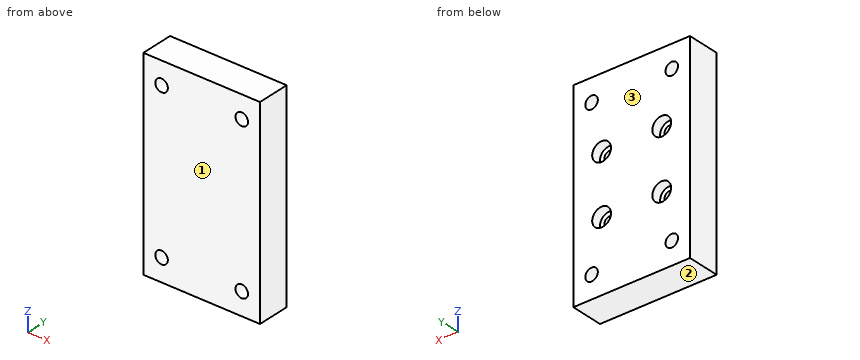
from build123d import *

# Parameters (mm, degrees)
SKETCH1_W                                       = 59.1185
SKETCH1_H                                       = 101.6
BOSS_EXTRUDE1_DEPTH                             = 16.51
CBORE_FOR_10_SOCKET_HEAD_CAP_SCREW1_D           = 5.1054
CBORE_FOR_10_SOCKET_HEAD_CAP_SCREW1_DEPTH       = 15.24
CBORE_FOR_10_SOCKET_HEAD_CAP_SCREW1_CBORE_D     = 9.525
CBORE_FOR_10_SOCKET_HEAD_CAP_SCREW1_CBORE_DEPTH = 4.826
F_1_4_0_25_DIAMETER_HOLE1_D                     = 6.35


with BuildPart() as part:
    # Sketch1 → Boss-Extrude1 (new body)
    with BuildSketch(Plane(origin=(0, 0, 0), x_dir=(1, 0, 0), z_dir=(0, 1, 0))):
        Rectangle(SKETCH1_W, SKETCH1_H)
    extrude(amount=BOSS_EXTRUDE1_DEPTH)

    # CBORE for #10 Socket Head Cap Screw1
    with Locations(Plane(origin=(-223.3968133, 16.51, 0), x_dir=(0, 0, 1), z_dir=(0, 1, 0))):
        with Locations((-14.986, 208.1568133), (14.986, 208.1568133), (14.986, 238.6368133), (-14.986, 238.6368133)):
            CounterBoreHole(CBORE_FOR_10_SOCKET_HEAD_CAP_SCREW1_D / 2, CBORE_FOR_10_SOCKET_HEAD_CAP_SCREW1_CBORE_D / 2, CBORE_FOR_10_SOCKET_HEAD_CAP_SCREW1_CBORE_DEPTH, depth=CBORE_FOR_10_SOCKET_HEAD_CAP_SCREW1_DEPTH)

    # 1/4 (0.25) Diameter Hole1 (through all)
    with Locations(Plane(origin=(0, 16.51, 0), x_dir=(1, 0, 0), z_dir=(0, 1, 0))):
        with Locations((20.32, -39.37), (-20.32, -39.37), (-20.32, 39.37), (20.32, 39.37)):
            Hole(F_1_4_0_25_DIAMETER_HOLE1_D / 2)


solid = part.part
Source: CAD feature listing. Evaluate the final solid. Frame: model axes, mm. Face numbers are marked on the shaded views. Give positions to 0.01 mm unless a question says otherwise; leave off trailing zeros. Order: outer loops, then holes, each group sorted by start corner. A loop starts at its lowest first (then second) coordinate and runs counter-clockwise, first axis right, second up. Notation, with made-up numbers: (46.25, 68.25) -> (100.25, 68.25) arc R27 cw to (100.25, 95.25) -> close; hole circle Ø4 at (36, 87.5). An arc over 180 degrees is marked (long way). Write item = value, one per line.
Item 1: Mould query, pull axis Y, two halves, no side actions, for the marked faces 1, 2 and 3. Classes: +Y half, -Y half, draft (parallel to the pull), parting line (faces both ways), or undercut.
Check result:
face_1 = -Y half
face_2 = draft
face_3 = +Y half
Item 2: Section query C-C (x = -21). Output: boundary loops of the cut face in (y, z), then the cut area to 3 significant figures.
Check result:
outline = (0, -50.8) -> (16.51, -50.8) -> (16.51, -42.47) -> (0, -42.47) -> close; (0, -36.27) -> (16.51, -36.27) -> (16.51, 36.27) -> (0, 36.27) -> close; (0, 42.47) -> (16.51, 42.47) -> (16.51, 50.8) -> (0, 50.8) -> close
area = 1,470 mm²
Item 3: Ray query, probe 1 along Z at (x, y) = (15, 8.5); probe 2 along X at (y, z) = (7, -39.37) (3 decimals); probe 3 along X at (y, z) = (14.25, -38.5). Return the intervals inside material, ascending.
Check result:
probe_1 = -50.8 to -17.53, -12.44 to 12.44, 17.53 to 50.8
probe_2 = -29.559 to -23.495, -17.145 to 17.145, 23.495 to 29.559
probe_3 = -29.56 to -23.37, -17.27 to 17.27, 23.37 to 29.56
Item 4: Section query A-A (y = 8.25). State how many separate pieces and enclosed holes the cut face has, then the cut area to 3 significant figures.
Check result:
separate_pieces = 1
enclosed_holes = 8
area = 5,800 mm²
Item 5: Contact query for flat-ended pins moving along their axis: pin 1 (5 mm diameter, centred on x = 13.5, z = -14, fed in from +Y); pin 2 (3 mm diameter, centred on x = -14.5, z = -15, fed in from +Y). Output: stop coordinate, or through.
Check result:
pin_1 = 11.68
pin_2 = 1.27
Item 6: Section query B-B (z = -39.37). Output: boundary loops of the cut face in (x, y) (3 decimals), then the cut area to 3 significant figures.
Check result:
outline = (-29.559, 0) -> (-23.495, 0) -> (-23.495, 16.51) -> (-29.559, 16.51) -> close; (-17.145, 0) -> (17.145, 0) -> (17.145, 16.51) -> (-17.145, 16.51) -> close; (23.495, 0) -> (29.559, 0) -> (29.559, 16.51) -> (23.495, 16.51) -> close
area = 766 mm²
